```python
from build123d import *

# Parameters (mm, degrees)
SKETCH1_R                  = 1.5
SKETCH1_W                  = 2.9
SKETCH1_H                  = 5
SKETCH1_W_2                = 6
SKETCH1_W_3                = 5
SKETCH1_H_2                = 22
BASE_FLANGE1_DEPTH         = 3
SKETCHED_START             = -31.946571622
SKETCHED_BEND1_DEPTH       = 45
SKETCHED_BEND1_2_OUTLINE_W = 3
SKETCHED_BEND1_2_OUTLINE_H = 16
SKETCHED_BEND1_2_DEPTH     = 45
SKETCHED_BEND1_3_OUTLINE_W = 3
SKETCHED_BEND1_3_OUTLINE_H = 5
SKETCHED_BEND1_3_DEPTH     = 16.5
SKETCHED_START_2           = 6.553428378
SKETCHED_BEND1_4_OUTLINE_W = 3
SKETCHED_BEND1_4_OUTLINE_H = 5
SKETCHED_BEND1_4_DEPTH     = 6.5
SKETCHED_START_3           = -49
SKETCHED_BEND1_5_OUTLINE_R = 1.5
SKETCHED_BEND1_5_DEPTH     = 98


with BuildPart() as part:
    # Base-Flange1: sheet metal written as solids
    # Sketch1 → Base-Flange1 (new body)
    with BuildSketch(Plane(origin=(0, 0, 0), x_dir=(1, 0, 0), z_dir=(0, 1, 0))):
        Polygon((-95, 31.946571622), (-95, -13.053428378), (95, -13.053428378), (95, 31.946571622), (45, 31.946571622), (-45, 31.946571622), align=None)
        with Locations(Location((92.5, -3.053428378, 0), (0, 0, 270))):
            Circle(SKETCH1_R, mode=Mode.SUBTRACT)
        with Locations(Location((92.5, 11.946571622, 0), (0, 0, 270))):
            Circle(SKETCH1_R, mode=Mode.SUBTRACT)
        with Locations(Location((-92.5, -3.053428378, 0), (0, 0, 90))):
            Circle(SKETCH1_R, mode=Mode.SUBTRACT)
        with Locations(Location((-92.5, 11.946571622, 0), (0, 0, 90))):
            Circle(SKETCH1_R, mode=Mode.SUBTRACT)
        with Locations((-39.45, 10.905641405)):
            Rectangle(SKETCH1_W, SKETCH1_H, mode=Mode.SUBTRACT)
        with Locations((-22.55, 22.947848405)):
            Rectangle(SKETCH1_W, SKETCH1_H, mode=Mode.SUBTRACT)
        with Locations((-31, 22.946571622)):
            Rectangle(SKETCH1_W_2, SKETCH1_H, mode=Mode.SUBTRACT)
        with Locations((-31, 10.946571622)):
            Rectangle(SKETCH1_W_2, SKETCH1_H, mode=Mode.SUBTRACT)
        with Locations((31, 10.946571622)):
            Rectangle(SKETCH1_W_2, SKETCH1_H, mode=Mode.SUBTRACT)
        with Locations((31, 22.946571622)):
            Rectangle(SKETCH1_W_2, SKETCH1_H, mode=Mode.SUBTRACT)
        with Locations((22.55, 22.947848405)):
            Rectangle(SKETCH1_W, SKETCH1_H, mode=Mode.SUBTRACT)
        with Locations((39.45, 10.905641405)):
            Rectangle(SKETCH1_W, SKETCH1_H, mode=Mode.SUBTRACT)
        with Locations((76.5, 4.446571622)):
            Rectangle(SKETCH1_W_3, SKETCH1_H_2, mode=Mode.SUBTRACT)
        with Locations((-76.5, 4.446571622)):
            Rectangle(SKETCH1_W_3, SKETCH1_H_2, mode=Mode.SUBTRACT)
    extrude(amount=-BASE_FLANGE1_DEPTH)

    # Sketched Bend1: read off the stored shape, not the designer's step
    # Sketched Bend1 outline → Sketched Bend1 (cut)
    with BuildSketch(Plane.XY.offset(SKETCHED_START)):
        with BuildLine():
            ThreePointArc((43.5, 0), (46.098076211, -0.825765386), (47.742640687, -3))
            Line((47.742640687, -3), (95, -3))
            Line((95, -3), (95, 0))
            Line((95, 0), (43.5, 0))
        make_face()
        with BuildLine():
            ThreePointArc((-47.742640687, -3), (-46.098076211, -0.825765386), (-43.5, 0))
            Line((-43.5, 0), (-95, 0))
            Line((-95, 0), (-95, -3))
            Line((-95, -3), (-47.742640687, -3))
        make_face()
    extrude(amount=SKETCHED_BEND1_DEPTH, mode=Mode.SUBTRACT)

    # Sketched Bend1 2 outline → Sketched Bend1 2 (add)
    with BuildSketch(Plane.XY.offset(SKETCHED_START)):
        with BuildLine():
            ThreePointArc((43.5, -3), (44.560660172, -3.439339828), (45, -4.5))
            Line((45, -4.5), (45, -32))
            Line((45, -32), (48, -32))
            Line((48, -32), (48, -4.5))
            ThreePointArc((48, -4.5), (47.935193518, -3.739041096), (47.742640687, -3))
            Line((47.742640687, -3), (43.5, -3))
        make_face()
        with BuildLine():
            ThreePointArc((-45, -4.5), (-44.560660172, -3.439339828), (-43.5, -3))
            Line((-43.5, -3), (-47.742640687, -3))
            ThreePointArc((-47.742640687, -3), (-47.935193518, -3.739041096), (-48, -4.5))
            Line((-48, -4.5), (-48, -32))
            Line((-48, -32), (-45, -32))
            Line((-45, -32), (-45, -4.5))
        make_face()
        with Locations((46.5, -45)):
            Rectangle(SKETCHED_BEND1_2_OUTLINE_W, SKETCHED_BEND1_2_OUTLINE_H)
        with Locations((-46.5, -45)):
            Rectangle(SKETCHED_BEND1_2_OUTLINE_W, SKETCHED_BEND1_2_OUTLINE_H)
    extrude(amount=SKETCHED_BEND1_2_DEPTH)

    # Sketched Bend1 3 outline → Sketched Bend1 3 (add)
    with BuildSketch(Plane.XY.offset(SKETCHED_START)):
        with Locations((46.5, -34.5)):
            Rectangle(SKETCHED_BEND1_3_OUTLINE_W, SKETCHED_BEND1_3_OUTLINE_H)
        with Locations((-46.5, -34.5)):
            Rectangle(SKETCHED_BEND1_3_OUTLINE_W, SKETCHED_BEND1_3_OUTLINE_H)
    extrude(amount=SKETCHED_BEND1_3_DEPTH)

    # Sketched Bend1 4 outline → Sketched Bend1 4 (add)
    with BuildSketch(Plane.XY.offset(SKETCHED_START_2)):
        with Locations((46.5, -34.5)):
            Rectangle(SKETCHED_BEND1_4_OUTLINE_W, SKETCHED_BEND1_4_OUTLINE_H)
        with Locations((-46.5, -34.5)):
            Rectangle(SKETCHED_BEND1_4_OUTLINE_W, SKETCHED_BEND1_4_OUTLINE_H)
    extrude(amount=SKETCHED_BEND1_4_DEPTH)

    # Sketched Bend1 5 outline → Sketched Bend1 5 (cut)
    with BuildSketch(Plane.YZ.offset(SKETCHED_START_3)):
        with Locations((-50.5, -11.946571622)):
            Circle(SKETCHED_BEND1_5_OUTLINE_R)
        with Locations((-50.5, 3.053428378)):
            Circle(SKETCHED_BEND1_5_OUTLINE_R)
    extrude(amount=SKETCHED_BEND1_5_DEPTH, mode=Mode.SUBTRACT)


solid = part.part
```
The model under review builds one solid part; all positions refer to its coordinate system, in mm. A direction names the side the tool comes from. Give positions to 0.01 mm unless a question says otherwise; leave off trailing zeros. Loops run counter-clockwise (first coordinate to the right, second up) from the corner with the lowest first, then second, coordinate; pieces in that order, holes last. Notation, with made-up numbers: (50.5, 4) -> (57.5, 4) arc R31 ccw to (57.5, 43) -> close; hole circle Ø11 at (71.5, 19.5). An arc over 180 degrees is marked (long way). Use CSV: the item, a comma, the result in double quotes.
1. Consider section C-C, the plane y = -50.5. Write out the cut boundary in (x, z).
Result:
outline,"(-48, -31.95) -> (-45, -31.95) -> (-45, -13.45) -> (-48, -13.45) -> close; (-48, -10.45) -> (-45, -10.45) -> (-45, 1.55) -> (-48, 1.55) -> close; (-48, 4.55) -> (-45, 4.55) -> (-45, 13.05) -> (-48, 13.05) -> close; (45, -31.95) -> (48, -31.95) -> (48, -13.45) -> (45, -13.45) -> close; (45, -10.45) -> (48, -10.45) -> (48, 1.55) -> (45, 1.55) -> close; (45, 4.55) -> (48, 4.55) -> (48, 13.05) -> (45, 13.05) -> close"
2. Consider section A-A, the plane z = 0. Write out the cut boundary in (x, y), then the cut area to 3 significant figures.
Result:
outline,"(-48, -53) -> (-45, -53) -> (-45, -37) -> (-48, -37) -> close; (-48, -32) -> (-45, -32) -> (-45, -4.5) arc R1.5 cw to (-43.5, -3) -> (43.5, -3) arc R1.5 cw to (45, -4.5) -> (45, -32) -> (48, -32) -> (48, -4.5) arc R4.5 ccw to (43.5, 0) -> (-43.5, 0) arc R4.5 ccw to (-48, -4.5) -> close; (45, -53) -> (48, -53) -> (48, -37) -> (45, -37) -> close"
area,"550 mm²"
3. For P1, Ø1.5, axis at y = -2, z = -23.5, coming from the -X side; P2, Ø2, axis at x = -35, z = -3.5, coming from the -Y side; P3, Ø0.9, axis at y = -2, z = -23.5, coming from the -X side; P4, Ø4, axis at x = -35.5, z = -18.5, coming from the +Y side, all flat-tipped, find the tip position at first contact; note any pin that passes through.
Result:
P1,"stops at x = -47.65"
P2,"stops at y = -3"
P3,"stops at x = -47.51"
P4,"stops at y = 0"
4. The part is to be moulded in two halves that separate along X. For faces 1 (the face through (-48, -28, -10)), 2 (the face through (-47, -34, 6.553)), 3 (the face through (-38, -1, -11)), say which applies: +X half, -X half, draft (parallel to the pull), parting line (faces both ways), or undercut.
Result:
face 1,"-X half"
face 2,"draft"
face 3,"undercut"
5. Consider section D-D, the plane y = -35. Write out the cut boundary in (x, z), then the cut area to 3 significant figures.
Result:
outline,"(-48, -31.95) -> (-45, -31.95) -> (-45, -15.45) -> (-48, -15.45) -> close; (-48, 6.55) -> (-45, 6.55) -> (-45, 13.05) -> (-48, 13.05) -> close; (45, -31.95) -> (48, -31.95) -> (48, -15.45) -> (45, -15.45) -> close; (45, 6.55) -> (48, 6.55) -> (48, 13.05) -> (45, 13.05) -> close"
area,"138 mm²"
6. To check wall thickness, follow probe 1 along Z at (x, y) = (-47.2, -50.5); probe 2 along X at (y, z) = (-17.5, -1.5); probe 3 along Z at (x, y) = (-46, -50). State the ranges of each line that lie inside material, in increasing order. Write a range as from..to.
Result:
probe 1,"z = -31.95..-13.45, -10.45..1.55, 4.55..13.05"
probe 2,"x = -48..-45, 45..48"
probe 3,"z = -31.95..-13.36, -10.53..1.64, 4.47..13.05"
7. Machinability: for faces 4 (the face through (-45, -29, -10)), 5 (the face through (46, -37, -5)), 6 (the face through (-39, -1, -13.406)), which of the approach directions +Z, -Z, +X, -X, +Y, -Y give a long, thin tool a straight path to every point of the face, cutting with its end or side? Answer none if there is none.
Result:
face 4,"+Z, -Z, -Y"
face 5,"+X, -X"
face 6,"+Y, -Y"
8. Consider section B-B, the plane y = -19. Write out the cut boundary in (x, z), then the cut area to 3 significant figures.
Result:
outline,"(-48, -31.95) -> (-45, -31.95) -> (-45, 13.05) -> (-48, 13.05) -> close; (45, -31.95) -> (48, -31.95) -> (48, 13.05) -> (45, 13.05) -> close"
area,"270 mm²"
